Read the model definition and answer for the solid it produces. Units are mm, in the model's axes. A direction names the side the tool comes from. Coordinates: 2 decimals unless noted, no trailing zeros. Loops run counter-clockwise (first coordinate to the right, second up) from the corner with the lowest first, then second, coordinate; pieces in that order, holes last.
from build123d import *

# Parameters (mm, degrees)
F0_W     = 40
F0_H     = 30
F1_DEPTH = 5
F2_W     = 20
F2_H     = 5
F3_DEPTH = 25
F4_W     = 5
F4_H     = 30
F5_DEPTH = 25
F6_W     = 5
F6_H     = 30
F7_DEPTH = 60
F8_W     = 35
F8_H     = 20
F9_DEPTH = 5


with BuildPart() as f1:
    # F0 (on Top) → F1 (new body)
    with BuildSketch(Plane.XY):
        with Locations((20, -15)):
            Rectangle(F0_W, F0_H)
    extrude(amount=F1_DEPTH)

    # F2 (on face) → F3 (join)
    with BuildSketch(Plane.XY.offset(5)):
        with Locations((10, -2.5)):
            Rectangle(F2_W, F2_H)
    extrude(amount=F3_DEPTH)

    # F4 (on face) → F5 (join)
    with BuildSketch(Plane.XY.offset(5)):
        with Locations((37.5, -15)):
            Rectangle(F4_W, F4_H)
    extrude(amount=F5_DEPTH)

    # F6 (on face) → F7 (join)
    with BuildSketch(Plane(origin=(0, 0, 0), x_dir=(-1, 0, 0), z_dir=(0, 1, 0))):
        with Locations((-37.5, 15)):
            Rectangle(F6_W, F6_H)
    extrude(amount=F7_DEPTH)

    # F8 (on face) → F9 (join)
    with BuildSketch(Plane(origin=(0, 0, 0), x_dir=(1, 0, 0), z_dir=(0, 0, -1))):
        with Locations((17.5, -50)):
            Rectangle(F8_W, F8_H)
    extrude(amount=-F9_DEPTH)


solid = f1.part
Item 1: A cutting plane is placed at B-B on x = 3.5. Determine the outline of the cut face in (y, z), then the cut area to 3 significant figures.
Numbers:
outline: (-30, 0) - (0, 0) - (0, 30) - (-5, 30) - (-5, 5) - (-30, 5) - close; (40, 0) - (60, 0) - (60, 5) - (40, 5) - close
area: 375 mm2
Item 2: A cutting plane is placed at A-A on z = 15. Determine the outline of the cut face in (x, y), then the cut area to 3 significant figures.
Numbers:
outline: (0, -5) - (20, -5) - (20, 0) - (0, 0) - close; (35, -30) - (40, -30) - (40, 60) - (35, 60) - close
area: 550 mm2
Item 3: A cutting plane is placed at C-C on y = 49.5. Determine the outline of the cut face in (x, z).
Numbers:
outline: (0, 0) - (40, 0) - (40, 30) - (35, 30) - (35, 5) - (0, 5) - close
Item 4: A cutting plane is placed at D-D on z = 2.5. Determine the outline of the cut face in (x, y).
Numbers:
outline: (0, -30) - (40, -30) - (40, 60) - (0, 60) - (0, 40) - (35, 40) - (35, 0) - (0, 0) - close
Item 5: Which of the six approach directions +Z, -Z, +X, -X, +Y, -Y give full straight-line access (tool end or side, diameter ignored) to faces 4 (the face through (0, -11, 3)), 5 (the face through (10, -5, 17)), 6 (the face through (17, 40, 2)), 7 (the face through (17, 50, 5)), 8 (the face through (20, -3, 17))?
Numbers:
face 4: +Z, -Z, -X, +Y, -Y
face 5: +Z, -X, -Y
face 6: +Z, -Z, -X
face 7: +Z, -X, +Y
face 8: +Z, +Y, -Y
Item 6: Determine the mould class of faces 1 (the face through (13, 0, 11)), 2 (the face through (23, -30, 4)), 3 (the face through (0, 50, 2)) for opening direction Y: released by +Y, released by -Y, zero draft, split by the parting line, or undercut.
Numbers:
face 1: undercut
face 2: released by -Y
face 3: zero draft
Item 7: Given pin 1 (2 mm diameter, centred on x = 19.5, z = 20.5, fed in from +Y); pin 2 (4 mm diameter, centred on y = 29.5, z = 7.5, fed in from -X); pin 3 (16 mm diameter, centred on x = 9, z = 19, fed in from -Y); pin 4 (24 mm diameter, centred on x = 25.5, y = -21, fed in from +Z), each flat-ended and moving along its own axis, determine where each tip first touches the part or whether it passes through.
Numbers:
pin 1: stops at y = 0
pin 2: stops at x = 35
pin 3: stops at y = -5
pin 4: stops at z = 30
Item 8: Find the intervals of material crossed by line 1 along Y through (x, z) = (14.5, 1.75); line 2 along Z through (x, y) = (28, -16.5); line 3 along Y through (x, z) = (13.5, 12.5), in increasing order.
Numbers:
line 1: y = -30 to 0, 40 to 60
line 2: z = 0 to 5
line 3: y = -5 to 0
